Here's how the part is built. I have some questions about the finished solid (model axes, mm). Face numbers are marked on the shaded views. A direction names the side the tool comes from. Give positions to 0.01 mm unless a question says otherwise; leave off trailing zeros. Write each loop counter-clockwise with the first axis right and the second up, starting at its lowest first coordinate (ties: lowest second). Pieces come first, ordered by that corner, then holes. Notation, with made-up numbers: (7, 61) - (15, 61) arc R30 ccw to (15, 89) - close; hole circle Ø11 at (57, 82). An arc over 180 degrees is marked (long way). Use one line per item in the form item = value. Start each with the question number.
from build123d import *

# Parameters (mm, degrees)
F0_W     = 544
F0_H     = 439
F1_DEPTH = 200
F2_R     = 20
F3_R     = 20
F4_T     = -10


with BuildPart() as f1:
    # F0 (on Top) → F1 (new body)
    with BuildSketch(Plane.XY):
        Rectangle(F0_W, F0_H)
    extrude(amount=F1_DEPTH)

    # F2
    f2_edges = [f1.edges().sort_by_distance(p)[0] for p in [
        (-272, -219.5, 100),
        (272, -219.5, 100),
        (272, 219.5, 100),
        (-272, 219.5, 100),
    ]]
    fillet(f2_edges, radius=F2_R)

    # F3
    f3_edges = [f1.edges().sort_by_distance(p)[0] for p in [
        (0, 219.5, 0),
    ]]
    fillet(f3_edges, radius=F3_R)

    # F4
    f4_openings = [f1.faces().sort_by_distance(p)[0] for p in [
        (0, 0, 200),
    ]]
    offset(amount=F4_T, openings=f4_openings)


solid = f1.part
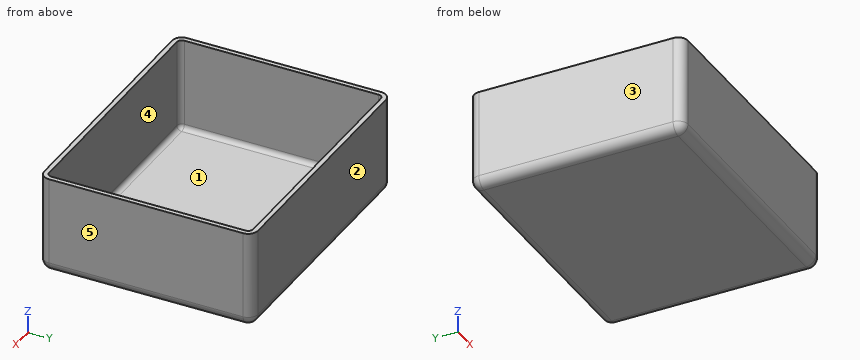
1. For P1, Ø10, axis at x = -138.5, y = -110, coming from the +Z side, with a flat end and sliding along its axis, tell me the tip position at first contact or that it passes through.
2. Please list where these lines run through material, in increasing order: line 1 (Y direction, x = -101, z = 170.5); line 2 (X direction, y = -191, z = 135.5); line 3 (Z direction, x = -138.5, y = -77).
3. We'd pull the mould along X, two halves only. Please class the marked faces 1, 2 and 3: pulls with the +X half, pulls with the -X half, needs draft (parallel to the pull), parting line crosses it, or undercut.
4. For the marked faces 4 and 5, which set-ups out of +Z, -Z, +X, -X, +Y, -Y let a thin tool reach every point of the face, with its end or its side?
5. I want a section at C-C, the plane y = 56. List the corners of the cut face in (x, z) for me.
6. I want a section at B-B, the plane x = 27.5. List the corners of the cut face in (y, z) for me.
7. I want a section at A-A, the plane z = 126. List the corners of the cut face in (x, y) for me, then the cut area to 3 significant figures.
Result sheet:
q1.P1 = 10
q2.line_1 = -219.5 to -209.5, 209.5 to 219.5
q2.line_2 = -272 to -262, 262 to 272
q2.line_3 = 0 to 10
q3.face_1 = undercut
q3.face_2 = needs draft
q3.face_3 = pulls with the -X half
q4.face_4 = +Z
q4.face_5 = +Z, -Z, +X, +Y, -Y
q5.outline = (-272, 20) arc R20 ccw to (-252, 0) - (252, 0) arc R20 ccw to (272, 20) - (272, 200) - (262, 200) - (262, 20) arc R10 cw to (252, 10) - (-252, 10) arc R10 cw to (-262, 20) - (-262, 200) - (-272, 200) - close
q6.outline = (-219.5, 20) arc R20 ccw to (-199.5, 0) - (199.5, 0) arc R20 ccw to (219.5, 20) - (219.5, 200) - (209.5, 200) - (209.5, 20) arc R10 cw to (199.5, 10) - (-199.5, 10) arc R10 cw to (-209.5, 20) - (-209.5, 200) - (-219.5, 200) - close
q7.outline = (-272, -199.5) arc R20 ccw to (-252, -219.5) - (252, -219.5) arc R20 ccw to (272, -199.5) - (272, 199.5) arc R20 ccw to (252, 219.5) - (-252, 219.5) arc R20 ccw to (-272, 199.5) - close; hole (-262, -199.5) arc R10 ccw to (-252, -209.5) - (252, -209.5) arc R10 ccw to (262, -199.5) - (262, 199.5) arc R10 ccw to (252, 209.5) - (-252, 209.5) arc R10 ccw to (-262, 199.5) - close
q7.area = 19,000 mm2
